Build history of the part. All positions in model axes, mm. A direction names the side the tool comes from. Give positions to 0.01 mm unless a question says otherwise; leave off trailing zeros. Write each loop counter-clockwise with the first axis right and the second up, starting at its lowest first coordinate (ties: lowest second). Pieces come first, ordered by that corner, then holes. Notation, with made-up numbers: (-0.5, 23) -> (15.5, 23) arc R25 cw to (15.5, 55) -> close; hole circle Ø9 at (59.5, -17.5). An arc over 180 degrees is marked (long way). Write item = value, one per line. Start each with the question number.
Q1. Wall check: line 1 (Y direction, x = -19.25, z = 3.6); line 2 (Y direction, x = 11, z = 3.75); line 3 (Y direction, x = 18, z = 1.1). Give the ranges that are in metal, low to high.
Q2. Saw through at A-A, the plane z = 5.4. List the corners of the cut face in (x, y).
Q3. Saw through at B-B, the plane x = 12.5. List the corners of the cut face in (y, z).
Q4. Saw through at C-C, the plane x = -19.25. List the corners of the cut face in (y, z).
Q5. Tool access for faces 4 (the face through (-13, 2.8, 3)), 5 (the face through (19, 10.15, 1)), 6 (the face through (-14, 5.3, 2)): list every direction of +Z, -Z, +X, -X, +Y, -Y with a clear straight run to the whole face (end or side of a thin tool).
Q6. Saw through at D-D, the plane y = -8. Give the number of separate pieces and of enclosed holes in the cut face, then the cut area to 3 significant figures.
Q7. Drop flat-ended pins along their axis: P1, Ø4.5, axis at x = -6, y = 8, coming from the -Z side; P2, Ø1.7, axis at x = 12, y = -1, coming from the +Z side; P3, Ø2, axis at x = -10, y = -5.5, coming from the +Z side. Give the stop position or say it passes through.
Q8. Mould opens along Y. For faces 1 (the face through (-4.7, 6.9, 6)), 2 (the face through (-17.1, -8, 1)), 3 (the face through (6.95, -8.5, 3.97)) say: pulls with the +Y half, pulls with the -Y half, needs draft (parallel to the pull), parting line crosses it, or undercut.
from build123d import *

# Parameters (mm, degrees)
SKETCH_W        = 44.5
SKETCH_H        = 22
SKETCH_R        = 1.75
SKETCH_R_2      = 1.3
PAD_DEPTH       = 4
SKETCH001_W     = 5.6
SKETCH001_H     = 5.6
POCKET_DEPTH    = 2
SKETCH002_W     = 4.3
SKETCH002_H     = 4.3
POCKET001_DEPTH = 2
SKETCH003_R     = 2.5
SKETCH003_R_2   = 1.3
PAD001_DEPTH    = 2
POCKET002_DEPTH = 4.001


with BuildPart() as part:
    # Sketch → Pad (new body)
    with BuildSketch(Plane.XY):
        Rectangle(SKETCH_W, SKETCH_H)
        with Locations((-12.5, 0)):
            Circle(SKETCH_R, mode=Mode.SUBTRACT)
        with Locations((12.5, 0)):
            Circle(SKETCH_R, mode=Mode.SUBTRACT)
        with Locations((-19.25, -8)):
            Circle(SKETCH_R_2, mode=Mode.SUBTRACT)
        with Locations((-5.75, 8)):
            Circle(SKETCH_R_2, mode=Mode.SUBTRACT)
        with Locations((19.25, 8)):
            Circle(SKETCH_R_2, mode=Mode.SUBTRACT)
        with Locations((5.75, -8)):
            Circle(SKETCH_R_2, mode=Mode.SUBTRACT)
    extrude(amount=PAD_DEPTH)

    # Sketch001 (on Face12 of Pad) → Pocket (cut)
    with BuildSketch(Plane.XY.offset(4)):
        with Locations((-12.5, 0)):
            Rectangle(SKETCH001_W, SKETCH001_H)
        with Locations((12.5, 0)):
            Rectangle(SKETCH001_W, SKETCH001_H)
    extrude(amount=-POCKET_DEPTH, mode=Mode.SUBTRACT)

    # Sketch002 → Pocket001 (cut)
    with BuildSketch(Plane(origin=(0, 0, 0), x_dir=(1, 0, 0), z_dir=(0, 0, -1))):
        with Locations((-19.25, 8)):
            Rectangle(SKETCH002_W, SKETCH002_H)
        with Locations((5.75, 8)):
            Rectangle(SKETCH002_W, SKETCH002_H)
        with Locations((-5.75, -8)):
            Rectangle(SKETCH002_W, SKETCH002_H)
        with Locations((19.25, -8)):
            Rectangle(SKETCH002_W, SKETCH002_H)
    extrude(amount=-POCKET001_DEPTH, mode=Mode.SUBTRACT)

    # Sketch003 (on Face5 of Pocket001) → Pad001 (join)
    with BuildSketch(Plane.XY.offset(4)):
        with Locations((-5.75, 8)):
            Circle(SKETCH003_R)
        with Locations((-5.75, 8)):
            Circle(SKETCH003_R_2, mode=Mode.SUBTRACT)
        with Locations((-19.25, -8)):
            Circle(SKETCH003_R)
        with Locations((-19.25, -8)):
            Circle(SKETCH003_R_2, mode=Mode.SUBTRACT)
        with Locations((5.75, -8)):
            Circle(SKETCH003_R)
        with Locations((5.75, -8)):
            Circle(SKETCH003_R_2, mode=Mode.SUBTRACT)
        with Locations((19.25, 8)):
            Circle(SKETCH003_R)
        with Locations((19.25, 8)):
            Circle(SKETCH003_R_2, mode=Mode.SUBTRACT)
    extrude(amount=PAD001_DEPTH)

    # Sketch004 (on Face5 of Pad001) → Pocket002 (cut, through all)
    with BuildSketch(Plane.XY.offset(4)):
        Polygon((-21.4, 10.15), (-10.4, 10.15), (-10.4, 5.3), (-17.8, 5.3), (-17.8, -3.35), (-21.4, -3.35), align=None)
        Polygon((17.8, 3.35), (21.4, 3.35), (21.4, -10.15), (10.4, -10.15), (10.4, -5.3), (17.8, -5.3), align=None)
        Polygon((-1.1, 10.15), (-1.1, 3.35), (-7.2, 3.35), (-7.2, 1.25), (7.2, 1.25), (7.2, 5.3), (15.3, 5.3), (15.3, 10.15), align=None)
        Polygon((-15.3, -5.3), (-15.3, -10.15), (1.1, -10.15), (1.1, -3.35), (7.2, -3.35), (7.2, -1.25), (-7.2, -1.25), (-7.2, -5.3), align=None)
    extrude(amount=-POCKET002_DEPTH, mode=Mode.SUBTRACT)


solid = part.part
Report:
q1.line_1 = -11 to -9.3, -6.7 to -3.35, 10.15 to 11
q1.line_2 = -11 to -10.15, -5.3 to -2.8, 2.8 to 5.3, 10.15 to 11
q1.line_3 = -11 to -10.15, 3.35 to 5.85, 10.15 to 11
q2.outline = circle Ø5 at (-19.25, -8); circle Ø5 at (-5.75, 8); circle Ø5 at (5.75, -8); circle Ø5 at (19.25, 8); hole circle Ø2.6 at (-19.25, -8); hole circle Ø2.6 at (-5.75, 8); hole circle Ø2.6 at (5.75, -8); hole circle Ø2.6 at (19.25, 8)
q3.outline = (-11, 0) -> (-10.15, 0) -> (-10.15, 4) -> (-11, 4) -> close; (-5.3, 0) -> (-1.75, 0) -> (-1.75, 2) -> (-2.8, 2) -> (-2.8, 4) -> (-5.3, 4) -> close; (1.75, 0) -> (5.3, 0) -> (5.3, 4) -> (2.8, 4) -> (2.8, 2) -> (1.75, 2) -> close; (10.15, 0) -> (11, 0) -> (11, 4) -> (10.15, 4) -> close
q4.outline = (-11, 0) -> (-10.15, 0) -> (-10.15, 2) -> (-9.3, 2) -> (-9.3, 6) -> (-10.5, 6) -> (-10.5, 4) -> (-11, 4) -> close; (-6.7, 2) -> (-5.85, 2) -> (-5.85, 0) -> (-3.35, 0) -> (-3.35, 4) -> (-5.5, 4) -> (-5.5, 6) -> (-6.7, 6) -> close; (10.15, 0) -> (11, 0) -> (11, 4) -> (10.15, 4) -> close
q5.face_4 = +Z
q5.face_5 = -Z
q5.face_6 = +Z, -Z
q6.separate_pieces = 5
q6.enclosed_holes = 0
q6.area = 50.4 mm2
q7.P1 = 0
q7.P2 = 2
q7.P3 = 4
q8.face_1 = needs draft
q8.face_2 = undercut
q8.face_3 = undercut
